Verification items for the finished model (mm, model axes). A direction names the side the tool comes from. Coordinates: 2 decimals unless noted, no trailing zeros. Write each loop counter-clockwise with the first axis right and the second up, starting at its lowest first coordinate (ties: lowest second). Pieces come first, ordered by that corner, then holes. Notation, with made-up numbers: M 58.5,46.25 L 98.5,46.25 A32 cw 98.5,81.25 Z; hole C -26,89 d11. An arc over 180 degrees is marked long. One line per item, written item: value.
```python
from build123d import *

# Parameters (mm, degrees)
SKETCH1_W            = 100
SKETCH1_H            = 75
BOSS_EXTRUDE1_DEPTH  = 1.5875
SKETCH2_W            = 20.53
SKETCH2_H            = 6
BOSS_EXTRUDE2_DEPTH  = 4.5875
LPATTERN1_COUNT      = 4
LPATTERN1_PITCH      = 24
LPATTERN1_COUNT_DIR2 = 2
LPATTERN1_PITCH_DIR2 = 25
SKETCH3_W            = 16.25
SKETCH3_H            = 4.25
BOSS_EXTRUDE3_DEPTH  = 4.45
LPATTERN2_COUNT      = 4
LPATTERN2_PITCH      = 24


with BuildPart() as part:
    # Sketch1 → Boss-Extrude1 (new body)
    with BuildSketch(Plane(origin=(0, 0, 0), x_dir=(1, 0, 0), z_dir=(0, 1, 0))):
        with Locations((50, 37.5)):
            Rectangle(SKETCH1_W, SKETCH1_H)
    extrude(amount=BOSS_EXTRUDE1_DEPTH)

    # Sketch2 → Boss-Extrude2 (add)
    with BuildSketch(Plane(origin=(0, 0, 0), x_dir=(1, 0, 0), z_dir=(0, 1, 0))):
        with Locations((13.985, 37.5)):
            Rectangle(SKETCH2_W, SKETCH2_H)
    boss_extrude2 = extrude(amount=BOSS_EXTRUDE2_DEPTH)

    # LPattern1: Boss-Extrude2 4 × 2
    with Locations(*[(i * LPATTERN1_PITCH, 0, -j * LPATTERN1_PITCH_DIR2) for i in range(LPATTERN1_COUNT) for j in range(LPATTERN1_COUNT_DIR2) if (i, j) != (0, 0)]):
        add(boss_extrude2)

    # Sketch3 → Boss-Extrude3 (add)
    with BuildSketch(Plane(origin=(0, 0, -75), x_dir=(-1, 0, 0), z_dir=(0, 0, -1))):
        with Locations((-13.875, 0.75)):
            Rectangle(SKETCH3_W, SKETCH3_H)
    boss_extrude3 = extrude(amount=BOSS_EXTRUDE3_DEPTH)

    # LPattern2: Boss-Extrude3 ×4
    with Locations(*[(i * LPATTERN2_PITCH, 0, 0) for i in range(1, LPATTERN2_COUNT)]):
        add(boss_extrude3)


solid = part.part
```
Item 1: Scan lines: line 1 (Z direction, x = 83, y = 1.9); line 2 (Z direction, x = 71, y = 3.3); line 3 (Y direction, x = 20, z = -31). Record each from-to range of solid material in increasing order.
The answers:
line 1: z = -79.45 to -75, -65.5 to -59.5, -40.5 to -34.5
line 2: z = -65.5 to -59.5, -40.5 to -34.5
line 3: y = 0 to 1.59
Item 2: Access from +Z, -Z, +X, -X, +Y, -Y to the whole of each face (thin tool, end or side, straight path). Record for faces 4 (the face through (48.25, 3, -62)), 5 (the face through (86, 3, -59.5)), 6 (the face through (86, 3, -34.5)).
The answers:
face 4: +Z, -Z, +Y
face 5: +X, -X, +Y
face 6: +Z, +X, -X, +Y
Item 3: Draft check along X on faces 1 (the face through (3.72, 3, -37)), 2 (the face through (14, 1, -79.45)), 3 (the face through (48.25, 3, -37)). Enter one of: released by +X, released by -X, zero draft, split by the parting line, or undercut.
The answers:
face 1: released by -X
face 2: zero draft
face 3: undercut
Item 4: Cross-section at A-A, the plane z = -63.5. Enter the section's corners in (x, y).
The answers:
outline: M 0,0 L 100,0 L 100,1.59 L 96.25,1.59 L 96.25,4.59 L 75.72,4.59 L 75.72,1.59 L 72.25,1.59 L 72.25,4.59 L 51.72,4.59 L 51.72,1.59 L 48.25,1.59 L 48.25,4.59 L 27.72,4.59 L 27.72,1.59 L 24.25,1.59 L 24.25,4.59 L 3.72,4.59 L 3.72,1.59 L 0,1.59 Z
Item 5: Cross-section at C-C, the plane z = -9. Enter the section's corners in (x, y), and give its area (3 significant figures).
The answers:
outline: M 0,0 L 100,0 L 100,1.59 L 0,1.59 Z
area: 159 mm²
Item 6: Go/stop test with flat-tipped pins: P1, Ø0.5, axis at x = 96.5, y = 0.5, coming from the -Z side; P2, Ø0.9, axis at y = 2.5, z = -36.5, coming from the -X side; P3, Ø1.3, axis at x = 15.5, z = -77.5, coming from the +Y side (3 decimals). Record where each tip stops, or that it passes through.
The answers:
P1: stops at z = -75
P2: stops at x = 3.72
P3: stops at y = 2.875
